Input: part model. Units: mm. Frame: model coordinates. A direction names the side the tool comes from. Coordinates: 2 decimals unless noted, no trailing zeros. Write each loop counter-clockwise with the first axis right and the second up, starting at its lowest first coordinate (ties: lowest second). Pieces come first, ordered by that corner, then holes.
from build123d import *

# Parameters (mm, degrees)
SKETCH_1_W      = 224
SKETCH_1_H      = 174
SKETCH_1_W_2    = 220
SKETCH_1_H_2    = 170
EXTRUDE_1_DEPTH = 32
SKETCH_2_W      = 227
SKETCH_2_H      = 177
SKETCH_2_W_2    = 217
SKETCH_2_H_2    = 167
EXTRUDE_2_DEPTH = 2
SKETCH_3_W      = 222
SKETCH_3_H      = 172
SKETCH_3_R      = 75
EXTRUDE_3_DEPTH = 2


with BuildPart() as part:
    # 草图1 → 凸台-拉伸1 (new body)
    with BuildSketch(Plane(origin=(0, 0, 0), x_dir=(1, 0, 0), z_dir=(0, 1, 0))):
        with Locations((110, -85)):
            Rectangle(SKETCH_1_W, SKETCH_1_H)
        with Locations((110, -85)):
            Rectangle(SKETCH_1_W_2, SKETCH_1_H_2, mode=Mode.SUBTRACT)
    extrude(amount=EXTRUDE_1_DEPTH)

    # 草图2 → 凸台-拉伸2 (add)
    with BuildSketch(Plane(origin=(0, 0, 0), x_dir=(1, 0, 0), z_dir=(0, 1, 0))):
        with Locations((110, -85)):
            Rectangle(SKETCH_2_W, SKETCH_2_H)
        with Locations((110, -85)):
            Rectangle(SKETCH_2_W_2, SKETCH_2_H_2, mode=Mode.SUBTRACT)
    extrude(amount=-EXTRUDE_2_DEPTH)

    # 草图3 → 凸台-拉伸3 (add)
    with BuildSketch(Plane(origin=(0, 32, 0), x_dir=(1, 0, 0), z_dir=(0, 1, 0))):
        with Locations((109, -84)):
            Rectangle(SKETCH_3_W, SKETCH_3_H)
        with Locations(Location((135, -78, 0), (0, 0, 270))):
            Circle(SKETCH_3_R, mode=Mode.SUBTRACT)
    extrude(amount=-EXTRUDE_3_DEPTH)


solid = part.part
Item 1: Access query for faces 4 (the face through (108, 16, 172)), 5 (the face through (220, 15, 86)), 6 (the face through (222, 16, 86)). Directions: +Z, -Z, +X, -X, +Y, -Y. A direction counts if a zero-diameter tool reaches every point of the face in a straight line with its end or side. Return the directions, or none.
Item 2: Material intervals for line 1 (X direction, y = 31.5, z = 78); line 2 (X direction, y = 29.5, z = 27); line 3 (Z direction, x = 32, y = 13), sorted ascending.
Item 3: Pull-direction query (X, two-part tool) for faces 1 (the face through (101, -2, 170)), 2 (the face through (-2, 16, 86)), 3 (the face through (209.362, 31.014, 68.236)); classes: released by +X, released by -X, zero draft, split by the parting line, or undercut.
Item 4: Section query C-C, the plane z = 78. Return loops of the section in (x, y).
Item 5: Section query D-D, the plane x = 24. Return loops of the section in (y, z).
Item 6: Section query B-B, the plane y = 3.5. Return loops of the section in (x, z).
Item 7: Section query A-A, the plane x = 135. Return loops of the section in (y, z), then the cut area to 3 significant figures.
Item 8: Pin query (flat end, axial travel): pin 1 Ø3 at (y, z) = (11, 54.5) entering from -X; pin 2 Ø4 at (x, y) = (35, 7.5) entering from +Z; pin 3 Ø4 at (x, y) = (64.5, 12) entering from -Z. Return the tip coordinate at first contact, or that it passes through.
The answers:
1. face 4: +Z, +X, -X, +Y
1. face 5: none
1. face 6: +Z, -Z, +X, +Y
2. line 1: x = -2 to 60, 210 to 222
2. line 2: x = -2 to 0, 220 to 222
2. line 3: z = -2 to 0, 170 to 172
3. face 1: zero draft
3. face 2: released by -X
3. face 3: undercut
4. outline: (-3.5, -2) - (1.5, -2) - (1.5, 0) - (0, 0) - (0, 30) - (60, 30) - (60, 32) - (-2, 32) - (-2, 0) - (-3.5, 0) - close; (210, 30) - (220, 30) - (220, 0) - (218.5, 0) - (218.5, -2) - (223.5, -2) - (223.5, 0) - (222, 0) - (222, 32) - (210, 32) - close
5. outline: (-2, -3.5) - (0, -3.5) - (0, -2) - (32, -2) - (32, 172) - (0, 172) - (0, 173.5) - (-2, 173.5) - (-2, 168.5) - (0, 168.5) - (0, 170) - (30, 170) - (30, 0) - (0, 0) - (0, 1.5) - (-2, 1.5) - close
6. outline: (-2, -2) - (222, -2) - (222, 172) - (-2, 172) - close; hole (0, 0) - (220, 0) - (220, 170) - (0, 170) - close
7. outline: (-2, -3.5) - (0, -3.5) - (0, -2) - (32, -2) - (32, 3) - (30, 3) - (30, 0) - (0, 0) - (0, 1.5) - (-2, 1.5) - close; (-2, 168.5) - (0, 168.5) - (0, 170) - (30, 170) - (30, 153) - (32, 153) - (32, 172) - (0, 172) - (0, 173.5) - (-2, 173.5) - close
7. area: 188 mm2
8. pin 1: stops at x = -2
8. pin 2: stops at z = 172
8. pin 3: stops at z = -2
